The listing builds one solid part. Answer for the finished solid, in the listing's coordinates (mm). Face numbers are marked on the shaded views. A direction names the side the tool comes from. Round coordinates to 2 decimals unless told otherwise and drop trailing zeros. Loops run counter-clockwise (first coordinate to the right, second up) from the corner with the lowest first, then second, coordinate; pieces in that order, holes last. Notation, with made-up numbers: (-11.75, 62) - (22.25, 62) arc R8 ccw to (22.25, 74) - close; hole circle Ø5 at (17.5, 40). An arc over 180 degrees is marked (long way). One line per item, written item: value.
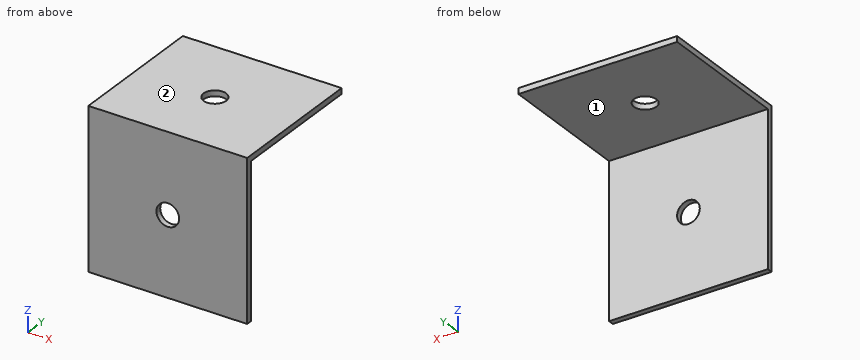
```python
from build123d import *

# Parameters (mm, degrees)
F0_W     = 88.9
F0_H     = 88.9
F1_DEPTH = 3.175
F2_W     = 88.9
F2_H     = 3.175
F3_DEPTH = 76.2
F4_R     = 6.35
F5_DEPTH = 3.175
F6_R     = 6.35
F7_DEPTH = 3.175


with BuildPart() as f1:
    # F0 (on Front) → F1 (new body)
    with BuildSketch(Plane.XZ):
        Rectangle(F0_W, F0_H)
    extrude(amount=F1_DEPTH)

    # F2 (on face) → F3 (join)
    with BuildSketch(Plane(origin=(0, 0, 0), x_dir=(-1, 0, 0), z_dir=(0, 1, 0))):
        with Locations((0, 42.8625)):
            Rectangle(F2_W, F2_H)
    extrude(amount=F3_DEPTH)

    # F4 (on face) → F5 (cut)
    with BuildSketch(Plane(origin=(0, 0, 0), x_dir=(-1, 0, 0), z_dir=(0, 1, 0))):
        Circle(F4_R)
    extrude(amount=-F5_DEPTH, mode=Mode.SUBTRACT)

    # F6 (on face) → F7 (cut)
    with BuildSketch(Plane.XY.offset(44.45)):
        with Locations((0, 36.406659)):
            Circle(F6_R)
    extrude(amount=-F7_DEPTH, mode=Mode.SUBTRACT)


solid = f1.part
```
1) Each of these flat-tipped pins is pushed along its axis until it touches: pin 1 Ø10 at (x, z) = (0, 0) entering from +Y; pin 2 Ø23 at (x, y) = (-13.5, 19.5) entering from -Z (3 decimals); pin 3 Ø8 at (x, z) = (28.5, 28.5) entering from +Y. Where does it stop, or does it pass through?
Final values:
pin 1: through
pin 2: z = 41.275
pin 3: y = 0
2) Consider L1, parallel to Z at x = 0, y = -1.8; L2, parallel to Y at x = 0, z = 42.5 (3 decimals); L3, parallel to Y at x = 1, z = 7 (3 decimals). Determine where each line is inside the solid, lowest interval first.
Final values:
L1: -44.45 to -6.35, 6.35 to 44.45
L2: -3.175 to 30.057, 42.757 to 76.2
L3: -3.175 to 0
3) A cutting plane is placed at B-B on z = 0. Give the vertices of the cut face in (x, y) (3 decimals).
Final values:
outline: (-44.45, -3.175) - (-6.35, -3.175) - (-6.35, 0) - (-44.45, 0) - close; (6.35, -3.175) - (44.45, -3.175) - (44.45, 0) - (6.35, 0) - close
4) A cutting plane is placed at D-D on y = 38. Give the vertices of the cut face in (x, z) (3 decimals), and give its area (3 significant figures).
Final values:
outline: (-44.45, 41.275) - (-6.147, 41.275) - (-6.147, 44.45) - (-44.45, 44.45) - close; (6.147, 41.275) - (44.45, 41.275) - (44.45, 44.45) - (6.147, 44.45) - close
area: 243 mm2
5) For the marked faces 1 and 2, determine the directions among +Z, -Z, +X, -X, +Y, -Y from which every point of the face is accessible in a straight line to the end or side of a thin tool.
Final values:
face 1: -Z, +X, -X, +Y
face 2: +Z, +X, -X, +Y, -Y
6) A cutting plane is placed at C-C on x = -31.5. Give the vertices of the cut face in (y, z) (3 decimals).
Final values:
outline: (-3.175, -44.45) - (0, -44.45) - (0, 41.275) - (76.2, 41.275) - (76.2, 44.45) - (-3.175, 44.45) - close
7) A cutting plane is placed at A-A on x = 0. Give the vertices of the cut face in (y, z) (3 decimals).
Final values:
outline: (-3.175, -44.45) - (0, -44.45) - (0, -6.35) - (-3.175, -6.35) - close; (-3.175, 6.35) - (0, 6.35) - (0, 41.275) - (30.057, 41.275) - (30.057, 44.45) - (-3.175, 44.45) - close; (42.757, 41.275) - (76.2, 41.275) - (76.2, 44.45) - (42.757, 44.45) - close
